Can you work these out from the model? Positions are in its coordinate system, mm. A direction names the side the tool comes from. Coordinates: 2 decimals unless noted, no trailing zeros. Write each loop counter-clockwise with the first axis right and the second up, starting at its lowest first coordinate (ties: lowest second). Pieces come first, ordered by that corner, then holes. Notation, with made-up numbers: (61, -23.75) - (68, -23.75) arc R15 cw to (68, 5.25) - close; hole circle Ø6 at (29.25, -21.75). An arc over 180 degrees is marked (long way). Use one line per item in the form item = value. Start each with the question number.
(1) If we section it at B-B on z = 8: Please give me the cut outline in (x, y).
(2) Thinking about a two-plate mould opening in X: for faces 1 (the face through (-4.523, 24, 11)), 2 (the face through (-92.288, -34.047, 11.59)), 3 (the face through (-76.3, 64.4, 24.7)), 4 (the face through (-3.759, 22.58, 24.676)), which applies, pulls with the +X half, pulls with the -X half, needs draft (parallel to the pull), parting line crosses it, or undercut?
(3) If we section it at A-A on y = -8: Please give me the cut outline in (x, z).
(4) If we section it at C-C on x = -34.5: Please give me the cut outline in (y, z).
(5) For pin 1 Ø1.5 at (x, z) = (-25.5, 22) entering from +Y, with a flat end and sliding along its axis, tell me the tip position at first contact or that it passes through.
(6) On a 3-axis mill with a long thin cutter (end or side, diameter ignored), from which of +Z, -Z, +X, -X, +Y, -Y can I reach the whole of each face in a straight line? I mean faces 5 (the face through (-59.143, 23, 11)), 6 (the face through (1.2, 64.4, 24.7)). Say none if no direction works.
(7) If I drill on probe 1 along X at (y, z) = (29, 12.5); probe 2 along Y at (x, z) = (-49.5, 12); probe 3 along X at (y, z) = (-13, 24), over which ranges is the centre line in solid material (lowest first)? Write a range as from..to.
```python
from build123d import *

# Parameters (mm, degrees)
F1_DEPTH = 25.4
F2_R     = 2.54
F3_R     = 2.54


with BuildPart() as f1:
    # F0 (on Top) → F1 (new body)
    with BuildSketch(Plane.XY):
        Polygon((-93.011853, 65.189209), (-93.011853, -34.810791), (6.988147, -34.810791), (6.988147, 65.189209), (-4.522704, 65.189209), (-4.522704, -18.92205), (-59.142936, -18.92205), (-59.142936, 65.189209), align=None)
    extrude(amount=F1_DEPTH)

    # F2
    f2_edges = [f1.edges().sort_by_distance(p)[0] for p in [
        (-93.011853, -34.810791, 12.7),
        (6.988147, -34.810791, 12.7),
        (-4.522704, -18.92205, 12.7),
        (-59.142936, -18.92205, 12.7),
        (-59.142936, 65.189209, 12.7),
        (-93.011853, 65.189209, 12.7),
        (6.988147, 65.189209, 12.7),
        (-4.522704, 65.189209, 12.7),
    ]]
    fillet(f2_edges, radius=F2_R)

    # F3
    f3_edges = [f1.edges().sort_by_distance(p)[0] for p in [
        (1.232722, 65.189209, 25.4),
        (6.244199, 64.445261, 25.4),
        (-3.778755, 64.445261, 25.4),
        (6.988147, 15.189209, 25.4),
        (-4.522704, 23.13358, 25.4),
        (6.244199, -34.066842, 25.4),
        (-5.266652, -18.178101, 25.4),
        (-43.011853, -34.810791, 25.4),
        (-31.83282, -18.92205, 25.4),
        (-92.267904, -34.066842, 25.4),
        (-58.398987, -18.178101, 25.4),
        (-93.011853, 15.189209, 25.4),
        (-59.142936, 23.13358, 25.4),
        (-92.267904, 64.445261, 25.4),
        (-59.886885, 64.445261, 25.4),
        (-76.077394, 65.189209, 25.4),
    ]]
    fillet(f3_edges, radius=F3_R)


solid = f1.part
```
Reported:
q1.outline = (-93.01, -32.27) arc R2.54 ccw to (-90.47, -34.81) - (4.45, -34.81) arc R2.54 ccw to (6.99, -32.27) - (6.99, 62.65) arc R2.54 ccw to (4.45, 65.19) - (-1.98, 65.19) arc R2.54 ccw to (-4.52, 62.65) - (-4.52, -16.38) arc R2.54 cw to (-7.06, -18.92) - (-56.6, -18.92) arc R2.54 cw to (-59.14, -16.38) - (-59.14, 62.65) arc R2.54 ccw to (-61.68, 65.19) - (-90.47, 65.19) arc R2.54 ccw to (-93.01, 62.65) - close
q2.face_1 = undercut
q2.face_2 = pulls with the -X half
q2.face_3 = needs draft
q2.face_4 = undercut
q3.outline = (-93.01, 0) - (-59.14, 0) - (-59.14, 22.86) arc R2.54 ccw to (-61.68, 25.4) - (-90.47, 25.4) arc R2.54 ccw to (-93.01, 22.86) - close; (-4.52, 0) - (6.99, 0) - (6.99, 22.86) arc R2.54 ccw to (4.45, 25.4) - (-1.98, 25.4) arc R2.54 ccw to (-4.52, 22.86) - close
q4.outline = (-34.81, 0) - (-18.92, 0) - (-18.92, 22.86) arc R2.54 ccw to (-21.46, 25.4) - (-32.27, 25.4) arc R2.54 ccw to (-34.81, 22.86) - close
q5.pin_1 = -18.92
q6.face_5 = +Z, -Z, +Y
q6.face_6 = +Z, +X, -X, +Y
q7.probe_1 = -93.01..-59.14, -4.52..6.99
q7.probe_2 = -34.81..-18.92
q7.probe_3 = -92.74..-59.41, -4.25..6.72
